```python
from build123d import *

# Parameters (mm, degrees)
CROQUIS1_R              = 10
SALIENTE_EXTRUIR1_DEPTH = 9
CHAFL_N1_SIZE           = 6.5
CHAFL_N1_SIZE2          = 4
SALIENTE_EXTRUIR3_DEPTH = 2.5
CROQUIS4_R              = 3
CORTAR_EXTRUIR1_DEPTH   = 186.864758197
CROQUIS5_R              = 3
CORTAR_EXTRUIR2_DEPTH   = 1
CROQUIS6_R              = 0.901496021
CORTAR_EXTRUIR3_DEPTH   = 16
SALIENTE_EXTRUIR4_DEPTH = 2.5


with BuildPart() as part:
    # Croquis1 → Saliente-Extruir1 (new body)
    with BuildSketch(Plane.XY):
        with Locations((-153.051797491, -38.56459666)):
            Circle(CROQUIS1_R)
    extrude(amount=SALIENTE_EXTRUIR1_DEPTH)

    # Chaflán1
    chafl_n1_edges = [part.edges().sort_by_distance(p)[0] for p in [
        (-163.051797491, -38.56459666, 9),
    ]]
    chafl_n1_side = [part.faces().sort_by_distance(p)[0] for p in [
        (-163.051797491, -38.56459666, 4.5),
    ]]
    chamfer(chafl_n1_edges, length=CHAFL_N1_SIZE, length2=CHAFL_N1_SIZE2, reference=chafl_n1_side[0])

    # Croquis3 → Saliente-Extruir3 (add)
    with BuildSketch(Plane(origin=(0, 0, 0), x_dir=(-1, 0, 0), z_dir=(0, 0, -1))):
        with BuildLine():
            Line((152.02722324, -41.384215004), (171.157627564, -48.335694708))
            ThreePointArc((171.157627564, -48.335694708), (178.428362583, -47.785764923), (173.206776067, -42.696458021))
            Line((173.206776067, -42.696458021), (154.076371743, -35.744978316))
            Line((154.076371743, -35.744978316), (152.02722324, -41.384215004))
        make_face()
    extrude(amount=-SALIENTE_EXTRUIR3_DEPTH)

    # Croquis4 → Cortar-Extruir1 (cut, through all)
    with BuildSketch(Plane.XY.offset(9)):
        with Locations((-153.051797491, -38.56459666)):
            Circle(CROQUIS4_R)
    extrude(amount=-CORTAR_EXTRUIR1_DEPTH, mode=Mode.SUBTRACT)

    # Croquis5 → Cortar-Extruir2 (cut)
    with BuildSketch(Plane.XY.offset(2.5)):
        with Locations((-174.668871458, -46.419665921)):
            Circle(CROQUIS5_R)
    extrude(amount=-CORTAR_EXTRUIR2_DEPTH, mode=Mode.SUBTRACT)

    # Croquis6 → Cortar-Extruir3 (cut)
    with BuildSketch(Plane.XY.offset(1.5)):
        with Locations((-174.668871458, -46.419665921)):
            Circle(CROQUIS6_R)
    extrude(amount=-CORTAR_EXTRUIR3_DEPTH, mode=Mode.SUBTRACT)

    # Croquis7 → Saliente-Extruir4 (add)
    with BuildSketch(Plane(origin=(0, 0, 0), x_dir=(-1, 0, 0), z_dir=(0, 0, -1))):
        with BuildLine():
            Line((142.472154892, -32.352593723), (144.077837211, -34.152336821))
            ThreePointArc((144.077837211, -34.152336821), (144.857254661, -32.833151134), (145.829058872, -31.648525027))
            Line((145.829058872, -31.648525027), (143.587737332, -30.757588058))
            ThreePointArc((143.587737332, -30.757588058), (142.398891813, -31.113717477), (142.472154892, -32.352593723))
        make_face()
        with BuildLine():
            Line((145.234815545, -29.108772462), (146.128114979, -31.349153467))
            ThreePointArc((146.128114979, -31.349153467), (147.223071886, -30.438960819), (148.436199285, -29.693505791))
            ThreePointArc((148.436199285, -29.693505791), (148.532872379, -29.643872708), (148.63007912, -29.595293084))
            Line((148.63007912, -29.595293084), (146.828644198, -27.991509074))
            ThreePointArc((146.828644198, -27.991509074), (145.589691401, -27.919552146), (145.234815545, -29.108772462))
        make_face()
        with BuildLine():
            Line((148.940319587, -27.005463152), (149.013491041, -29.416259051))
            ThreePointArc((149.013491041, -29.416259051), (150.353718186, -28.935455054), (151.748645686, -28.649870472))
            ThreePointArc((151.748645686, -28.649870472), (151.856464194, -28.636294775), (151.964423861, -28.623891525))
            Line((151.964423861, -28.623891525), (150.820155195, -26.500700496))
            ThreePointArc((150.820155195, -26.500700496), (149.680531113, -26.009336288), (148.940319587, -27.005463152))
        make_face()
        with BuildLine():
            ThreePointArc((155.218271428, -28.802097457), (155.324230846, -28.826216577), (155.42992191, -28.851485714))
            Line((155.42992191, -28.851485714), (155.080835189, -26.464975839))
            ThreePointArc((155.080835189, -26.464975839), (154.177995305, -25.613470127), (153.141728543, -26.296355938))
            Line((153.141728543, -26.296355938), (152.38594646, -28.586789165))
            ThreePointArc((152.38594646, -28.586789165), (153.366736356, -28.569557215), (154.344495765, -28.648502108))
            ThreePointArc((154.344495765, -28.648502108), (154.783087756, -28.715605137), (155.218271428, -28.802097457))
        make_face()
        with BuildLine():
            ThreePointArc((158.426588439, -30.131825925), (158.517908498, -30.190730739), (158.608583057, -30.250624434))
            Line((158.608583057, -30.250624434), (159.09678329, -27.888644024))
            ThreePointArc((159.09678329, -27.888644024), (158.53962342, -26.779700963), (157.332290487, -27.066979615))
            Line((157.332290487, -27.066979615), (155.83871334, -28.96079012))
            ThreePointArc((155.83871334, -28.96079012), (156.766248042, -29.280047284), (157.6580406, -29.688644631))
            ThreePointArc((157.6580406, -29.688644631), (158.047231669, -29.901708148), (158.426588439, -30.131825925))
        make_face()
        with BuildLine():
            ThreePointArc((160.986626339, -32.478670998), (161.052292491, -32.565256717), (161.117013855, -32.652550905))
            Line((161.117013855, -32.652550905), (162.38361689, -30.599989658))
            ThreePointArc((162.38361689, -30.599989658), (162.239338735, -29.367364148), (161.006561803, -29.224385594))
            Line((161.006561803, -29.224385594), (158.955337038, -30.493151881))
            ThreePointArc((158.955337038, -30.493151881), (159.717742172, -31.110391034), (160.416004535, -31.799357964))
            ThreePointArc((160.416004535, -31.799357964), (160.708852496, -32.132683364), (160.986626339, -32.478670998))
        make_face()
        with BuildLine():
            ThreePointArc((162.589606773, -35.559568525), (162.621698713, -35.663391632), (162.652660529, -35.767557347))
            Line((162.652660529, -35.767557347), (164.544895347, -34.271984441))
            ThreePointArc((164.544895347, -34.271984441), (164.830900984, -33.06434931), (163.721371142, -32.508358875))
            Line((163.721371142, -32.508358875), (161.35990674, -32.999049004))
            ThreePointArc((161.35990674, -32.999049004), (161.865224995, -33.839821995), (162.285736417, -34.726058929))
            ThreePointArc((162.285736417, -34.726058929), (162.446919484, -35.139442249), (162.589606773, -35.559568525))
        make_face()
    extrude(amount=-SALIENTE_EXTRUIR4_DEPTH)


solid = part.part
```
Source: CAD feature listing. Evaluate the final solid. Frame: model axes, mm. A direction names the side the tool comes from. Round coordinates to 2 decimals unless told otherwise and drop trailing zeros. Write each loop counter-clockwise with the first axis right and the second up, starting at its lowest first coordinate (ties: lowest second). Pieces come first, ordered by that corner, then holes. Notation, with made-up numbers: M -34.75,83.5 L -7.75,83.5 A26 cw -7.75,110.5 Z; hole C 85,-27.75 d11. An arc over 180 degrees is marked long. Use CSV: the item, a comma, the result in double quotes. Start each with the question number.
Q1. Pull-direction query (Y, two-part tool) for faces 1 (the face through (-144, -32, 2.5)), 2 (the face through (-171.807, -45.519, 2.007)), 3 (the face through (-147.742, -28.805, 1.232)), 4 (the face through (-143.264, -33.24, 1.232)); classes: +Y half, -Y half, draft (parallel to the pull), parting line (faces both ways), or undercut.
Q2. Access query for faces 5 (the face through (-151.4, -27.58, 1.23)), 6 (the face through (-161, -30, 2.5)), 7 (the face through (-156, -40, 9)). Directions: +Z, -Z, +X, -X, +Y, -Y. A direction counts if a zero-diameter tool reaches every point of the face in a straight line with its end or side. Return the directions, or none.
Q3. Cut plane D-D on z = 3.5. Output: boundary loops of the cut face in (x, y), plus the area to 3 significant figures.
Q4. Cut plane C-C on x = -172.5. Output: boundary loops of the cut face in (y, z).
Q5. Cut plane A-A on z = 1. Count the separate pieces of the cut face and the enclosed holes in it, plus the area to 3 significant figures.
Q6. First-contact query: P1, Ø2.5, axis at x = -158, y = -28, coming from the +Z side; P2, Ø3, axis at x = -160.5, y = -31.5, coming from the +Z side; P3, Ø3.5, axis at x = -174.67, y = -46.42, coming from the +Z side. Flat tips, straight axial feed; report the tip coordinate or a pass-through.
Q7. Cut plane B-B on z = 7. Output: boundary loops of the cut face in (x, y).
Q8. Line query: line 1 (X direction, y = -28, z = 1); line 2 (X direction, y = -38.5, z = 3.5); line 3 (Y direction, x = -162, z = 1.25). Output: solid intervals per line, ascending. Write a range as from..to.
Results found:
1,face 1,"draft"
1,face 2,"undercut"
1,face 3,"+Y half"
1,face 4,"undercut"
2,face 5,"+Z, -Z, +Y"
2,face 6,"+Z, -X, +Y"
2,face 7,"+Z, +X, -X, +Y, -Y"
3,outline,"C -153.05,-38.56 d18.77; hole C -153.05,-38.56 d6"
3,area,"248 mm^2"
4,outline,"M -49.78,0 L -42.44,0 L -42.44,2.5 L -44.35,2.5 L -44.35,1.5 L -48.49,1.5 L -48.49,2.5 L -49.78,2.5 Z"
5,separate pieces,"1"
5,enclosed holes,"2"
5,area,"438 mm^2"
6,P1,"z = 2.5"
6,P2,"z = 4.51"
6,P3,"z = 1.5"
7,outline,"C -153.05,-38.56 d14.46; hole C -153.05,-38.56 d6"
8,line 1,"-159.07..-156.6, -155.31..-152.58, -151.63..-148.97, -146.84..-145.49"
8,line 2,"-162.44..-156.05, -150.05..-143.67"
8,line 3,"-45.01..-32.87, -31.22..-29.19"
